CAD build for the part. Positions are in the model's coordinates, mm. Round coordinates to 2 decimals unless told otherwise and drop trailing zeros. Loops run counter-clockwise (first coordinate to the right, second up) from the corner with the lowest first, then second, coordinate; pieces in that order, holes last. Notation, with made-up numbers: M 56,49 L 112,49 A12 ccw 112,65 Z; hole C -30.5,-26.75 d2. An arc over 180 degrees is marked long. Use a Markdown table: item, result. Add a question column.
(1) Wall check: L1, parallel to Y at x = 827.5, z = 20.5; L2, parallel to Z at x = 791.5, y = -34.5. Give the ranges that are in metal, low to high.
(2) Band-saw the part on B-B, the plane z = 19.5. Write the cut outline in (x, y).
(3) Flat gauge pins, fed straight in: P1, Ø5, axis at x = 417, z = 14.5, coming from the -Y side; P2, Ø5, axis at x = 568, z = 19, coming from the -Y side; P3, Ø9.5, axis at x = 358.5, y = -35.5, coming from the +Z side. Where does each tip first touch, or does it go through?
(4) Band-saw the part on A-A, the plane x = -59. Write the cut outline in (y, z).
from build123d import *

# Parameters (mm, degrees)
F0_W      = 1270
F0_H      = 82.55
F1_DEPTH  = 12.7
F0_H_2    = 19.05
F1_FACE_W = 1270
F1_FACE_H = 82.55
F2_DEPTH  = 12.7


with BuildPart() as f1:
    # F0 (on Top) → F1 (new body)
    with BuildSketch(Plane.XY):
        with Locations((378.964252, 18.430763)):
            Rectangle(F0_W, F0_H)
    extrude(amount=F1_DEPTH)

    # F0 (on Top) + F1_face (on face) → F2 (join)
    with BuildSketch(Plane.XY):
        with Locations((378.964252, 18.430763)):
            Rectangle(F0_W, F0_H)
        with Locations((378.964252, -32.369237)):
            Rectangle(F0_W, F0_H_2)
    with BuildSketch(Plane(origin=(378.964252, 18.430763, 12.7), x_dir=(1, 0, 0), z_dir=(0, 0, 1))):
        Rectangle(F1_FACE_W, F1_FACE_H)
    extrude(amount=F2_DEPTH)


solid = f1.part
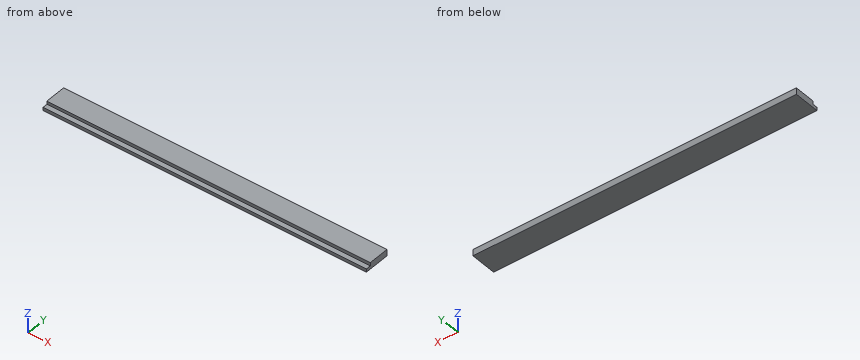
Return value:
| question | item | result |
|---|---|---|
| 1 | L1 | -22.84 to 59.71 |
| 1 | L2 | 0 to 12.7 |
| 2 | outline | M -256.04,-22.84 L 1013.96,-22.84 L 1013.96,59.71 L -256.04,59.71 Z |
| 3 | P1 | y = -41.89 |
| 3 | P2 | y = -22.84 |
| 3 | P3 | z = 12.7 |
| 4 | outline | M -41.89,0 L 59.71,0 L 59.71,25.4 L -22.84,25.4 L -22.84,12.7 L -41.89,12.7 Z |
